Part model, mm, in its own coordinate system. Give positions to 0.01 mm unless a question says otherwise; leave off trailing zeros. Write each loop counter-clockwise with the first axis right and the second up, starting at its lowest first coordinate (ties: lowest second). Pieces come first, ordered by that corner, then holes. Notation, with made-up numbers: (89, 26) - (134, 26) arc R9 cw to (134, 36) - close; hole circle Ø5 at (6, -9). An arc over 180 degrees is marked (long way). Answer in a Markdown table with one row per item. Add a question column.
1. Band-saw the part on C-C on x = -28. Write the cut outline in (y, z) (1 decimal), plus the area to 3 significant figures.
2. Probe line 1 along X through (y, z) = (1.8, 0); line 2 along Z through (x, y) = (45.5, 2.3); line 3 along X through (y, z) = (0.3, 0.5). List the from-to ranges inside material, lowest first.
3. Band-saw the part on D-D on x = 52. Write the cut outline in (y, z) (3 decimals).
4. Band-saw the part on A-A on z = 0. Write the cut outline in (x, y) (3 decimals), plus the area to 3 significant figures.
5. Drop flat-ended pins along their axis: pin 1 Ø6 at (x, z) = (-13, -2) entering from -Y; pin 2 Ø1.5 at (y, z) = (1.5, 2.5) entering from +X. Give the stop position or say it passes through.
6. Band-saw the part on B-B on y = 2.35. State how many separate pieces and enclosed holes the cut face has, plus the area to 3 significant figures.
```python
from build123d import *

# Parameters (mm, degrees)
SKETCH1_R           = 3.175
SKETCH1_R_2         = 1.905
BOSS_EXTRUDE1_DEPTH = 3.175
FILLET1_R           = 12.7


with BuildPart() as part:
    # Sketch1 → Boss-Extrude1 (new body)
    with BuildSketch(Plane(origin=(0, 0, 0), x_dir=(1, 0, 0), z_dir=(0, 1, 0))):
        with BuildLine():
            ThreePointArc((-57.050749937, 4.875846131), (-67.466363723, -0.174069026), (-56.789646398, -4.645574453))
            Line((-56.789646398, -4.645574453), (42.161094502, -1.93207299))
            ThreePointArc((42.161094502, -1.93207299), (51.000262943, -2.46173496), (59.613169718, -4.518255666))
            ThreePointArc((59.613169718, -4.518255666), (65.637005666, -1.505580282), (62.624330282, 4.518255666))
            ThreePointArc((62.624330282, 4.518255666), (52.396503486, 6.960374005), (41.899990962, 7.589347594))
            Line((41.899990962, 7.589347594), (-57.050749937, 4.875846131))
        make_face()
        with Locations((-61.11875, 0)):
            Circle(SKETCH1_R, mode=Mode.SUBTRACT)
        with Locations((61.11875, 0)):
            Circle(SKETCH1_R_2, mode=Mode.SUBTRACT)
    extrude(amount=BOSS_EXTRUDE1_DEPTH)

    # Fillet1
    fillet1_edges = [part.edges().sort_by_distance(p)[0] for p in [
        (-56.789646398, 1.5875, 4.645574453),
        (-57.050749937, 1.5875, -4.875846131),
    ]]
    fillet(fillet1_edges, radius=FILLET1_R)


solid = part.part
```
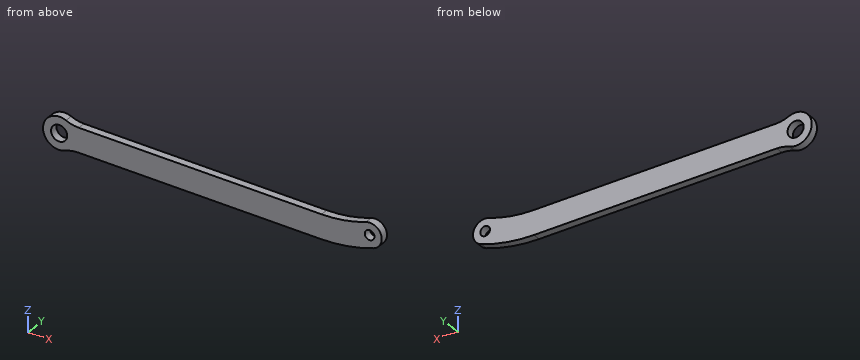
Values:
| question | item | result |
|---|---|---|
| 1 | outline | (0, -5.7) - (3.2, -5.7) - (3.2, 3.9) - (0, 3.9) - close |
| 1 | area | 30.3 mm² |
| 2 | line 1 | x = -67.47 to -64.29, -57.94 to 59.21, 63.02 to 65.88 |
| 2 | line 2 | z = -7.58 to 1.95 |
| 2 | line 3 | x = -67.45 to -64.25, -57.98 to 59.28, 62.96 to 65.85 |
| 3 | outline | (0, -7.018) - (3.175, -7.018) - (3.175, 2.62) - (0, 2.62) - close |
| 4 | outline | (-67.469, 0) - (-64.294, 0) - (-64.294, 3.175) - (-67.469, 3.175) - close; (-57.944, 0) - (59.214, 0) - (59.214, 3.175) - (-57.944, 3.175) - close; (63.024, 0) - (65.881, 0) - (65.881, 3.175) - (63.024, 3.175) - close |
| 4 | area | 391 mm² |
| 5 | pin 1 | stops at y = 0 |
| 5 | pin 2 | stops at x = 65.55 |
| 6 | separate pieces | 1 |
| 6 | enclosed holes | 2 |
| 6 | area | 1,230 mm² |
